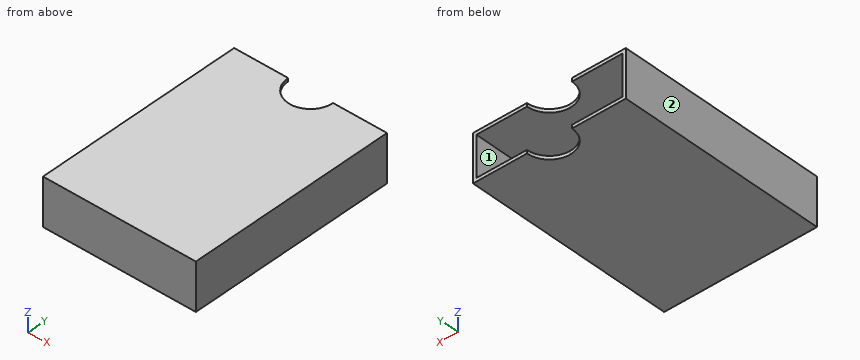
from build123d import *

# Parameters (mm, degrees)
SKETCH1_W           = 68
SKETCH1_H           = 21
SKETCH1_W_2         = 65
SKETCH1_H_2         = 18
BOSS_EXTRUDE1_DEPTH = 1.5
SKETCH2_W           = 68
SKETCH2_H           = 21
SKETCH2_W_2         = 65
SKETCH2_H_2         = 18
BOSS_EXTRUDE2_DEPTH = 92
CUT_EXTRUDE1_REACH  = 103.682


with BuildPart() as part:
    # Sketch1 → Boss-Extrude1 (new body)
    # profile 1 of 2: a face of its own
    with BuildSketch(Plane(origin=(0, 0, 0), x_dir=(1, 0, 0), z_dir=(0, 1, 0))):
        Rectangle(SKETCH1_W, SKETCH1_H)
        Rectangle(SKETCH1_W_2, SKETCH1_H_2, mode=Mode.SUBTRACT)
    # profile 2 of 2: a face of its own
    with BuildSketch(Plane(origin=(0, 0, 0), x_dir=(1, 0, 0), z_dir=(0, 1, 0))):
        Rectangle(SKETCH1_W_2, SKETCH1_H_2)
    extrude(amount=BOSS_EXTRUDE1_DEPTH)

    # Sketch2 → Boss-Extrude2 (add)
    with BuildSketch(Plane(origin=(0, 1.5, 0), x_dir=(1, 0, 0), z_dir=(0, 1, 0))):
        Rectangle(SKETCH2_W, SKETCH2_H)
        Rectangle(SKETCH2_W_2, SKETCH2_H_2, mode=Mode.SUBTRACT)
    extrude(amount=BOSS_EXTRUDE2_DEPTH)

    # Cut-Extrude1: up to this face of the body (flat: up to its plane)
    cut_extrude1_end = Plane(part.part.faces().sort_by_distance((0, 46.75, -10.5))[0])
    # Sketch3 → Cut-Extrude1 (cut, up to the picked face)
    with BuildSketch(Plane.XY.offset(10.5), mode=Mode.PRIVATE) as cut_extrude1_sk1:
        with BuildLine():
            Line((10, 93.5), (0, 93.5))
            Line((0, 93.5), (0, 83.5))
            ThreePointArc((0, 83.5), (7.071067812, 86.428932188), (10, 93.5))
        make_face()
    cut_extrude1_tool1 = split(extrude(cut_extrude1_sk1.sketch, amount=-CUT_EXTRUDE1_REACH, mode=Mode.PRIVATE), bisect_by=cut_extrude1_end, keep=Keep.BOTH, mode=Mode.PRIVATE)
    # Sketch3 → Cut-Extrude1 (cut, up to the picked face)
    with BuildSketch(Plane.XY.offset(10.5), mode=Mode.PRIVATE) as cut_extrude1_sk2:
        with BuildLine():
            Line((0, 83.5), (0, 93.5))
            Line((0, 93.5), (-10, 93.5))
            ThreePointArc((-10, 93.5), (-7.071067812, 86.428932188), (0, 83.5))
        make_face()
    cut_extrude1_tool2 = split(extrude(cut_extrude1_sk2.sketch, amount=-CUT_EXTRUDE1_REACH, mode=Mode.PRIVATE), bisect_by=cut_extrude1_end, keep=Keep.BOTH, mode=Mode.PRIVATE)
    # Sketch3 → Cut-Extrude1 (cut, up to the picked face)
    with BuildSketch(Plane.XY.offset(10.5), mode=Mode.PRIVATE) as cut_extrude1_sk3:
        with BuildLine():
            Line((10, 93.5), (0, 93.5))
            Line((0, 93.5), (0, 83.5))
            ThreePointArc((0, 83.5), (7.071067812, 86.428932188), (10, 93.5))
        make_face()
    cut_extrude1_tool3 = split(extrude(cut_extrude1_sk3.sketch, amount=-CUT_EXTRUDE1_REACH, mode=Mode.PRIVATE), bisect_by=cut_extrude1_end, keep=Keep.BOTH, mode=Mode.PRIVATE)
    # Sketch3 → Cut-Extrude1 (cut, up to the picked face)
    with BuildSketch(Plane.XY.offset(10.5), mode=Mode.PRIVATE) as cut_extrude1_sk4:
        with BuildLine():
            Line((0, 83.5), (0, 93.5))
            Line((0, 93.5), (-10, 93.5))
            ThreePointArc((-10, 93.5), (-7.071067812, 86.428932188), (0, 83.5))
        make_face()
    cut_extrude1_tool4 = split(extrude(cut_extrude1_sk4.sketch, amount=-CUT_EXTRUDE1_REACH, mode=Mode.PRIVATE), bisect_by=cut_extrude1_end, keep=Keep.BOTH, mode=Mode.PRIVATE)
    add(cut_extrude1_tool1.solids().sort_by(Axis((4.244132, 89.255868, 10.5), (0, 0, -1)))[0], mode=Mode.SUBTRACT)
    add(cut_extrude1_tool2.solids().sort_by(Axis((-4.244132, 89.255868, 10.5), (0, 0, -1)))[0], mode=Mode.SUBTRACT)
    add(cut_extrude1_tool3.solids().sort_by(Axis((4.244132, 89.255868, 10.5), (0, 0, -1)))[0], mode=Mode.SUBTRACT)
    add(cut_extrude1_tool4.solids().sort_by(Axis((-4.244132, 89.255868, 10.5), (0, 0, -1)))[0], mode=Mode.SUBTRACT)


solid = part.part
Source: CAD feature listing. Evaluate the final solid. Frame: model axes, mm. Face numbers are marked on the shaded views. A direction names the side the tool comes from. Coordinates: 2 decimals unless noted, no trailing zeros. Order: outer loops, then holes, each group sorted by start corner. A loop starts at its lowest first (then second) coordinate and runs counter-clockwise, first axis right, second up. Notation, with made-up numbers: M 1.25,-2 L 40.25,-2 A11 ccw 40.25,16 Z; hole C -8.5,68 d9. An arc over 180 degrees is marked long. Write each question's results on one line, items separated by ' | '. Start each with the question number.
Item 1: Cut plane C-C (z = 1.75). Return loops of the section in (x, y), and give its area (3 significant figures).
Item 2: Cut plane B-B (x = -14.5). Return loops of the section in (y, z).
Item 3: First-contact query: pin 1 Ø10 at (x, z) = (-5, 5) entering from -Y; pin 2 Ø6 at (x, z) = (-8, -4) entering from +Y. Flat tips, straight axial feed; report the tip coordinate or a pass-through.
Item 4: Line query: probe 1 along X at (y, z) = (51, 0); probe 2 along Z at (x, y) = (30.5, 54.5); probe 3 along Y at (x, z) = (6, 0.75). Output: solid intervals per line, ascending.
Item 5: Cut plane A-A (y = 21). Return loops of the section in (x, z), and give its area (3 significant figures).
Item 6: Set-up query: the marked faces 1 and 2. Return all of +Z, -Z, +X, -X, +Y, -Y with unobstructed straight access to the full face (end or side cutting, diameter ignored); none if empty.
Checked values:
1) outline: M -34,0 L 34,0 L 34,93.5 L 32.5,93.5 L 32.5,1.5 L -32.5,1.5 L -32.5,93.5 L -34,93.5 Z | area: 378 mm2
2) outline: M 0,-10.5 L 93.5,-10.5 L 93.5,-9 L 1.5,-9 L 1.5,9 L 93.5,9 L 93.5,10.5 L 0,10.5 Z
3) pin 1: stops at y = 0 | pin 2: stops at y = 1.5
4) probe 1: x = -34 to -32.5, 32.5 to 34 | probe 2: z = -10.5 to -9, 9 to 10.5 | probe 3: y = 0 to 1.5
5) outline: M -34,-10.5 L 34,-10.5 L 34,10.5 L -34,10.5 Z; hole M -32.5,-9 L 32.5,-9 L 32.5,9 L -32.5,9 Z | area: 258 mm2
6) face 1: +Y | face 2: +Z, -Z, -X, +Y, -Y
